Read the model definition and answer for the solid it produces. Units are mm, in the model's axes. A direction names the side the tool comes from. Coordinates: 2 decimals unless noted, no trailing zeros. Order: outer loops, then holes, each group sorted by start corner. A loop starts at its lowest first (then second) coordinate and runs counter-clockwise, first axis right, second up. Notation, with made-up numbers: (-18.75, 66) - (24.25, 66) arc R21 cw to (24.25, 88) - close; hole circle Ø8 at (62.25, 78.25). An arc over 180 degrees is marked (long way). Write item = value, one per line.
from build123d import *

# Parameters (mm, degrees)
EXTRUDE_1_DEPTH             = 10
HOLE_WIZARD_2_5_2_5_1_D     = 2.5
HOLE_WIZARD_2_5_2_5_1_DEPTH = 15
HOLE_WIZARD_2_5_2_5_2_D     = 2.5
HOLE_WIZARD_2_5_2_5_2_DEPTH = 15


with BuildPart() as part:
    # 草圖1 → 填料-伸長1 (new body)
    with BuildSketch(Plane(origin=(0, 0, -5), x_dir=(-1, 0, 0), z_dir=(0, 0, -1))):
        Polygon((-7.5, 0), (7.5, 0), (7.5, 3), (-4.5, 3), (-4.5, 15), (-7.5, 15), align=None)
    extrude(amount=-EXTRUDE_1_DEPTH)

    # Ø2.5 (2.5) 直徑孔1
    with Locations(Plane(origin=(7.5, 0, 0), x_dir=(0, 0, -1), z_dir=(1, 0, 0))):
        with Locations((0, 10)):
            Hole(HOLE_WIZARD_2_5_2_5_1_D / 2, depth=HOLE_WIZARD_2_5_2_5_1_DEPTH)

    # Ø2.5 (2.5) 直徑孔2
    with Locations(Plane(origin=(0, 0, 0), x_dir=(-1, 0, 0), z_dir=(0, -1, 0))):
        with Locations((2.5, 0)):
            Hole(HOLE_WIZARD_2_5_2_5_2_D / 2, depth=HOLE_WIZARD_2_5_2_5_2_DEPTH)


solid = part.part
1) The part is cut by section A-A (z = 0.75). Determine the outline of the cut face in (x, y), and give its area (3 significant figures).
Returned:
outline = (-7.5, 0) - (-3.5, 0) - (-3.5, 3) - (-7.5, 3) - close; (-1.5, 0) - (7.5, 0) - (7.5, 9) - (4.5, 9) - (4.5, 3) - (-1.5, 3) - close; (4.5, 11) - (7.5, 11) - (7.5, 15) - (4.5, 15) - close
area = 69.0 mm^2
2) The part is cut by section D-D (z = -2.75). Determine the outline of the cut face in (x, y), and give its area (3 significant figures).
Returned:
outline = (-7.5, 0) - (7.5, 0) - (7.5, 15) - (4.5, 15) - (4.5, 3) - (-7.5, 3) - close
area = 81.0 mm^2
3) A flat-ended cylindrical pin translates along its axis: pin 1 Ø1 at (x, z) = (-4, 1) entering from +Y. Find the tip coordinate at first contact, or state that the pin passes through.
Returned:
pin_1 = 3
4) Straight lines are drawn through the part: line 1 along Y through (x, z) = (6.9, 0); line 2 along X through (y, z) = (11.75, -0.25); line 3 along Y through (x, z) = (1.5, -0.5). For each, find the intervals that lie inside material, in ascending order. Write a range as from..to.
Returned:
line_1 = 0..8.75, 11.25..15
line_2 = 4.5..7.5
line_3 = 0..3
5) The part is cut by section C-C (x = -2.5). Determine the outline of the cut face in (y, z), and give its area (3 significant figures).
Returned:
outline = (0, -5) - (3, -5) - (3, -1.25) - (0, -1.25) - close; (0, 1.25) - (3, 1.25) - (3, 5) - (0, 5) - close
area = 22.5 mm^2
6) The part is cut by section B-B (y = 10.75). Determine the outline of the cut face in (x, z), and give its area (3 significant figures).
Returned:
outline = (4.5, -5) - (7.5, -5) - (7.5, -1) - (4.5, -1) - close; (4.5, 1) - (7.5, 1) - (7.5, 5) - (4.5, 5) - close
area = 24.0 mm^2
7) Determine the mould class of faces 3 (the face through (5.98, 11.24, -0.16)), 4 (the face through (6, 15, 0)), 5 (the face through (-1.31, 1.52, -0.38)), 6 (the face through (0, 0, 0)) for opening direction Y: pulls with the +Y half, pulls with the -Y half, needs draft (parallel to the pull), parting line crosses it, or undercut.
Returned:
face_3 = undercut
face_4 = pulls with the +Y half
face_5 = needs draft
face_6 = pulls with the -Y half
8) For faces 1 (the face through (-7.5, 1, 0)), 2 (the face through (4.5, 9, -1)), determine the directions among +Z, -Z, +X, -X, +Y, -Y from which every point of the face is accessible in a straight line to the end or side of a thin tool.
Returned:
face_1 = +Z, -Z, -X, +Y, -Y
face_2 = +Z, -Z, -X, +Y
